Autodesk Inventor part; units mm, degrees
ref_plane "YZ Plane" through (0, 0, 0) normal (1, 0, 0) x (0, 1, 0)
ref_plane "XZ Plane" through (0, 0, 0) normal (0, 1, 0) x (-1, 0, 0)
ref_plane "XY Plane" through (0, 0, 0) normal (0, 0, 1) x (1, 0, 0)
sketch "スケッチ1" plane through (0, 0, 0) normal (1, 0, 0) x (0, 1, 0)
  line L0 (0, 0) -> (1.6, 0)
  line L1 (1.6, 0) -> (1.6, 2.5)
  line L2 (1.6, 2.5) -> (4.6, 2.5)
  line L3 (4.6, 2.5) -> (4.6, -9.5)
  line L4 (4.6, -9.5) -> (1.6, -9.5)
  line L5 (1.6, -9.5) -> (1.6, -7)
  line L6 (1.6, -7) -> (0, -7)
  line L7 (0, -7) -> (0, 0)
  dimension "d0" = 4.6
  dimension "d1" = 7
  dimension "d2" = 12
  dimension "d3" = 2.5
  dimension "d4" = 3
extrude "押し出し1" add sketch "スケッチ1" along normal blind 20
sketch "スケッチ2" plane through (0, 0, -7) normal (0, -1, 0) x (1, 0, 0)
  circle A0 centre (5, 3.5) radius 1.5
  circle A1 centre (15, 3.5) radius 1.5
  line L0 (0, 0) -> (0, 7)
  point P0 (0, 3.5)
  dimension "d7" = 3
  dimension "d8" = 3
  dimension "d9" = 5
  dimension "d10" = 10
extrude "押し出し2" cut sketch "スケッチ2" against normal through all
properties part number "slider2b" material "アルミニウム 6061-AHC"
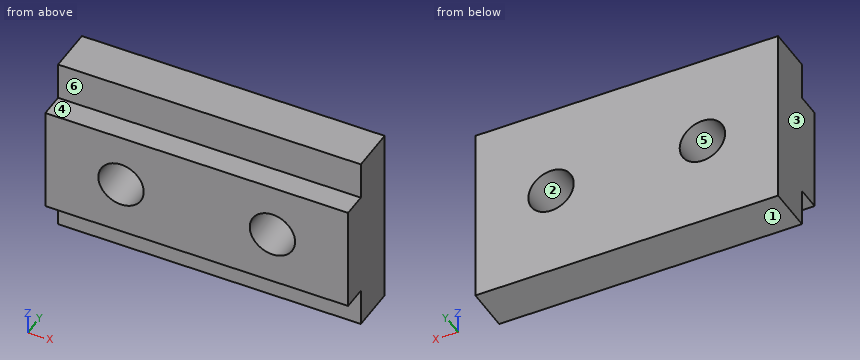
Verification items for the finished model (mm, model axes). Face numbers are marked on the shaded views. A direction names the side the tool comes from. Coordinates: 2 decimals unless noted, no trailing zeros. Write each loop counter-clockwise with the first axis right and the second up, starting at its lowest first coordinate (ties: lowest second). Pieces come first, ordered by that corner, then holes. Notation, with made-up numbers: (25.5, -28) -> (71.5, -28) arc R14 ccw to (71.5, -9) -> close; hole circle Ø11 at (76.25, -34). An arc over 180 degrees is marked (long way). One line per item, written item: value. Start each with the question number.
Q1. Mould release check, pull along Z, two halves, no side actions. Record for the marked faces 1, 2, 3 and 4: pulls with the +Z half, pulls with the -Z half, needs draft (parallel to the pull), parting line crosses it, or undercut.
Q2. Cross-section at D-D on x = 18.25. Enter the section's corners in (y, z).
Q3. Cross-section at B-B on z = -3.5. Enter the section's corners in (x, y).
Q4. Thickness scan on L1, parallel to Z at x = 15, y = 1.7; L2, parallel to Z at x = 15, y = 0.75; L3, parallel to X at y = 3.95, z = -4. Record the ranges inside material, lowest first. Write a range as from..to.
Q5. Cross-section at A-A on x = 15. Enter the section's corners in (y, z), and give its area (3 significant figures).
Q6. Go/stop test with flat-tipped pins: P1, Ø0.5, axis at x = 14.5, y = 1, coming from the -Z side; P2, Ø1.2, axis at x = 8, z = 1, coming from the -Y side; P3, Ø1.3, axis at x = 8.5, y = 0.5, coming from the +Z side. Record where each tip stops, or that it passes through.
Q7. Access from +Z, -Z, +X, -X, +Y, -Y to the whole of each face (thin tool, end or side, straight path). Record for the marked faces 5 and 6.
Q8. Cross-section at C-C on y = 1.15. Enter the section's corners in (x, z).
Checked values:
1. face 1: pulls with the -Z half
1. face 2: undercut
1. face 3: needs draft
1. face 4: pulls with the +Z half
2. outline: (0, -7) -> (1.6, -7) -> (1.6, -9.5) -> (4.6, -9.5) -> (4.6, 2.5) -> (1.6, 2.5) -> (1.6, 0) -> (0, 0) -> close
3. outline: (0, 0) -> (3.5, 0) -> (3.5, 4.6) -> (0, 4.6) -> close; (6.5, 0) -> (13.5, 0) -> (13.5, 4.6) -> (6.5, 4.6) -> close; (16.5, 0) -> (20, 0) -> (20, 4.6) -> (16.5, 4.6) -> close
4. L1: z = -9.5..-5, -2..2.5
4. L2: z = -7..-5, -2..0
4. L3: x = 0..3.59, 6.41..13.59, 16.41..20
5. outline: (0, -7) -> (1.6, -7) -> (1.6, -9.5) -> (4.6, -9.5) -> (4.6, -5) -> (0, -5) -> close; (0, -2) -> (4.6, -2) -> (4.6, 2.5) -> (1.6, 2.5) -> (1.6, 0) -> (0, 0) -> close
5. area: 33.4 mm²
6. P1: stops at z = -7
6. P2: stops at y = 1.6
6. P3: stops at z = 0
7. face 5: +Y, -Y
7. face 6: +Z, +X, -X, -Y
8. outline: (0, -7) -> (20, -7) -> (20, 0) -> (0, 0) -> close; hole circle Ø3 at (5, -3.5); hole circle Ø3 at (15, -3.5)
